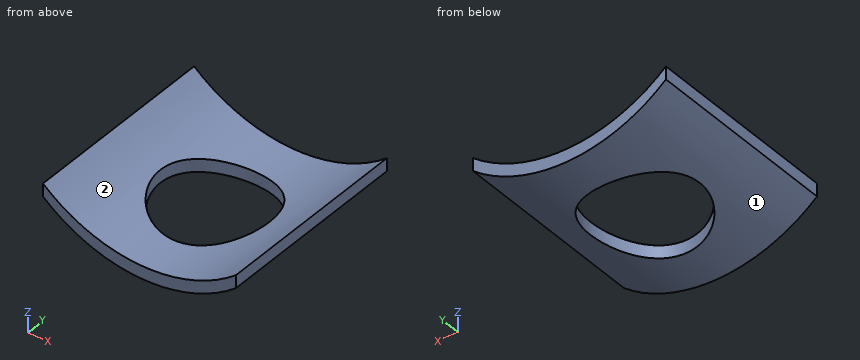
```python
from build123d import *

# Parameters (mm, degrees)
PAD_DEPTH    = 225
SKETCH001_R  = 127.5
POCKET_DEPTH = 111.905868


with BuildPart() as part:
    # Sketch → Pad (new body, symmetric)
    with BuildSketch(Plane.XZ):
        with BuildLine():
            ThreePointArc((-225, 111.904868), (0, 30), (225, 111.904868))
            Line((225, 111.904868), (225, 81.904868))
            ThreePointArc((-225, 81.904868), (0, 0), (225, 81.904868))
            Line((-225, 111.904868), (-225, 81.904868))
        make_face()
    extrude(amount=PAD_DEPTH, both=True)

    # Sketch001 → Pocket (cut, through all)
    with BuildSketch(Plane.XY):
        Circle(SKETCH001_R)
    extrude(amount=POCKET_DEPTH, mode=Mode.SUBTRACT)


solid = part.part
```
Check sheet for the modelled part. Datum: model origin and axes. Units: mm. Face numbers are marked on the shaded views. Give positions to 0.01 mm unless a question says otherwise; leave off trailing zeros. Order: outer loops, then holes, each group sorted by start corner. A loop starts at its lowest first (then second) coordinate and runs counter-clockwise, first axis right, second up. Notation, with made-up numbers: (15, 80) -> (21, 80) arc R13 ccw to (21, 87) -> close; hole circle Ø2 at (-31.75, -1). An arc over 180 degrees is marked (long way). Use CSV: the item, a comma, the result in double quotes. Start each with the question number.
1) Sectioned sample at A-A, the plane x = 0. Record the boundary of the cut face in (y, z), plus the area to 3 significant figures.
2) Sectioned sample at B-B, the plane y = -22. Record the boundary of the cut face in (x, z).
3) Go/stop test with flat-tipped pins: P1, Ø6, axis at y = 86, z = 65.5, coming from the +X side (3 decimals); P2, Ø6, axis at y = 129.5, z = 33.5, coming from the +X side. Record where each tip stops, or that it passes through.
4) Sectioned sample at C-C, the plane z = 46. Record the boundary of the cut face in (x, y), plus the area to 3 significant figures.
5) Material ranges on line 1 (X direction, y = -187, z = 88.5); line 2 (X direction, y = -192, z = 73.5); line 3 (Y direction, x = 0, z = 14), recorded low to high. Write a range as from..to.
6) Mould release check, pull along X, two halves, no side actions. Record for the marked faces 1 and 2: released by +X, released by -X, zero draft, split by the parting line, or undercut.
Recorded:
1,outline,"(-225, 0) -> (-127.5, 0) -> (-127.5, 30) -> (-225, 30) -> close; (127.5, 0) -> (225, 0) -> (225, 30) -> (127.5, 30) -> close"
1,area,"5,850 mm2"
2,outline,"(-225, 81.9) arc R350 ccw to (-125.59, 23.31) -> (-125.59, 53.31) arc R350 cw to (-225, 111.9) -> close; (125.59, 23.31) arc R350 ccw to (225, 81.9) -> (225, 111.9) arc R350 cw to (125.59, 53.31) -> close"
3,P1,"x = 207.985"
3,P2,"x = 155.62"
4,outline,"(-173.45, -225) -> (-104.61, -225) -> (-104.61, -72.89) arc R127.5 cw to (-104.61, 72.89) -> (-104.61, 225) -> (-173.45, 225) -> close; (104.61, -225) -> (173.45, -225) -> (173.45, 225) -> (104.61, 225) -> (104.61, 72.89) arc R127.5 cw to (104.61, -72.89) -> close"
4,area,"57,400 mm2"
5,line 1,"-225..-193.72, 193.72..225"
5,line 2,"-214.59..-168.99, 168.99..214.59"
5,line 3,"-225..-127.5, 127.5..225"
6,face 1,"split by the parting line"
6,face 2,"undercut"
